Input: part model. Units: mm. Frame: model coordinates. Face numbers are marked on the shaded views. A direction names the side the tool comes from. Give positions to 0.01 mm unless a question says otherwise; leave off trailing zeros. Loops run counter-clockwise (first coordinate to the right, second up) from the corner with the lowest first, then second, coordinate; pieces in that order, holes last. Notation, with made-up numbers: M -11,83 L 47,83 A22 ccw 47,98 Z; hole C 26,-14.75 d1. An arc over 180 degrees is marked long. Answer as a JSON object with one key per item and string values. Group by question number.
1) First-contact query: P1, Ø2, axis at x = -1.5, z = -1, coming from the +Y side; P2, Ø2, axis at y = 5.5, z = 0.5, coming from the -X side; P3, Ø1, axis at y = 0.5, z = -0.5, coming from the +X side. Flat tips, straight axial feed; report the tip coordinate or a pass-through.
2) Section query A-A on x = 0. Return loops of the section in (y, z).
3) Ray query, L1, parallel to Y at x = -0.35, z = 1.45; L2, parallel to Y at x = -1.05, z = -0.65; L3, parallel to Z at x = -0.65, y = 3. Return the intervals inside material, ascending.
4) Section query C-C on z = 0. Return loops of the section in (x, y).
5) Section query B-B on z = 1.3. Return loops of the section in (x, y), plus the area to 3 significant figures.
6) Section query D-D on y = 2. Return loops of the section in (x, z).
7) Draft query along Y for the marked faces 3, 4 and 5. Return one class per face: +Y half, -Y half, draft (parallel to the pull), parting line (faces both ways), or undercut.
8) Access query for the marked faces 1 and 2. Directions: +Z, -Z, +X, -X, +Y, -Y. A direction counts if a zero-diameter tool reaches every point of the face in a straight line with its end or side. Return the directions, or none.
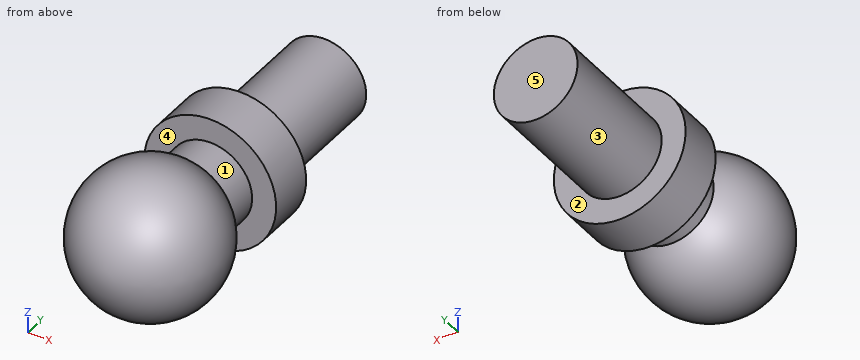
from build123d import *

# Parameters (mm, degrees)
SKETCH4_R      = 1.1303
EXTRUDE1_DEPTH = 7.366
SKETCH5_R      = 1.778
EXTRUDE2_DEPTH = 1.27


with BuildPart() as part:
    # Sketch3 → Revolve1 (revolve)
    with BuildSketch(Plane.XY):
        with BuildLine():
            Line((0, 1.9685), (0, -1.9685))
            ThreePointArc((0, -1.9685), (1.9685, 0), (0, 1.9685))
        make_face()
    revolve(axis=Axis((0, 1.9685, 0), (0, -1, 0)))

    # Sketch4 → Extrude1 (add)
    with BuildSketch(Plane(origin=(0, 0, 0), x_dir=(-1, 0, 0), z_dir=(0, 1, 0))):
        Circle(SKETCH4_R)
    extrude(amount=EXTRUDE1_DEPTH)

    # Sketch5 → Extrude2 (add)
    with BuildSketch(Plane(origin=(0, 2.54, 0), x_dir=(-1, 0, 0), z_dir=(0, 1, 0))):
        Circle(SKETCH5_R)
    extrude(amount=EXTRUDE2_DEPTH)


solid = part.part
Output:
{
 "1": {"P1": "stops at y = 7.37", "P2": "stops at x = -1.13", "P3": "stops at x = 1.96"},
 "2": {"outline": "M 1.61,-1.13 L 2.54,-1.13 L 2.54,-1.78 L 3.81,-1.78 L 3.81,-1.13 L 7.37,-1.13 L 7.37,1.13 L 3.81,1.13 L 3.81,1.78 L 2.54,1.78 L 2.54,1.13 L 1.61,1.13 A1.97 ccw long Z"},
 "3": {"L1": "y = -1.28 to 1.28, 2.54 to 3.81", "L2": "y = -1.53 to 1.53, 2.54 to 3.81", "L3": "z = -1.65 to 1.65"},
 "4": {"outline": "M -1.78,2.54 L -1.13,2.54 L -1.13,1.61 A1.97 ccw long 1.13,1.61 L 1.13,2.54 L 1.78,2.54 L 1.78,3.81 L 1.13,3.81 L 1.13,7.37 L -1.13,7.37 L -1.13,3.81 L -1.78,3.81 Z"},
 "5": {"outline": "C 0,0 d2.96; M -1.21,2.54 L 1.21,2.54 L 1.21,3.81 L -1.21,3.81 Z", "area": "9.95 mm^2"},
 "6": {"outline": "C 0,0 d2.26"},
 "7": {"face 3": "draft", "face 4": "undercut", "face 5": "+Y half"},
 "8": {"face 1": "none", "face 2": "+Y"}
}
